```python
from build123d import *

# Parameters (mm, degrees)
AUFSATZ_LINEAR_AUSTRAGEN1_DEPTH = 25
VERRUNDUNG1_R                   = 0.2


with BuildPart() as part:
    # Skizze1 → Aufsatz-Linear austragen1 (new body)
    with BuildSketch(Plane.XY):
        Polygon((2.95, 2), (1, 2), (1, 0), (0, 0), (0, 2.79), (0.25, 2.79), (0.25, 3.01), (0, 3.01), (0, 5.8), (1, 5.8), (1, 3.8), (2.95, 3.8), align=None)
    extrude(amount=AUFSATZ_LINEAR_AUSTRAGEN1_DEPTH)

    # Verrundung1
    verrundung1_edges = [part.edges().sort_by_distance(p)[0] for p in [
        (0.5, 5.8, 0),
        (1, 4.8, 0),
        (0.25, 2.9, 25),
        (1.975, 3.8, 0),
        (2.95, 2.9, 0),
        (1.975, 2, 0),
        (1, 1, 0),
        (0.5, 0, 0),
        (0, 1.395, 0),
        (0.125, 2.79, 0),
        (0.25, 2.9, 0),
        (0.125, 3.01, 0),
        (0, 4.405, 0),
        (0.125, 2.79, 25),
        (0, 5.8, 12.5),
        (1, 5.8, 12.5),
        (0, 1.395, 25),
        (2.95, 3.8, 12.5),
        (2.95, 2, 12.5),
        (1, 0, 12.5),
        (0, 0, 12.5),
        (0.5, 0, 25),
        (1, 1, 25),
        (1.975, 2, 25),
        (2.95, 2.9, 25),
        (1.975, 3.8, 25),
        (1, 4.8, 25),
        (0.5, 5.8, 25),
        (0, 4.405, 25),
        (0.125, 3.01, 25),
    ]]
    fillet(verrundung1_edges, radius=VERRUNDUNG1_R)


solid = part.part
```
Geometry check sheet. Reference: the model listing, model coordinates, mm. A direction names the side the tool comes from. Give positions to 0.01 mm unless a question says otherwise; leave off trailing zeros. Write each loop counter-clockwise with the first axis right and the second up, starting at its lowest first coordinate (ties: lowest second). Pieces come first, ordered by that corner, then holes. Notation, with made-up numbers: (79.5, -15) -> (115.5, -15) arc R24 ccw to (115.5, -2) -> close; hole circle Ø1 at (75, 87). An arc over 180 degrees is marked (long way). Use one line per item in the form item = value.
Item 1: Access from +Z, -Z, +X, -X, +Y, -Y to the whole of each face (thin tool, end or side, straight path). Record for faces 1 (the flat face through (2.95, 3, 12)), 2 (the flat face through (1, 5, 12)), 3 (the flat face through (2, 2, 12)).
Results list:
face_1 = +Z, -Z, +X, +Y, -Y
face_2 = +Z, -Z, +X, +Y
face_3 = +Z, -Z, +X, -Y
Item 2: Depth check by flat-ended pin: pin 1 Ø0.9 at (x, z) = (2, 7.5) entering from -Y; pin 2 Ø2 at (y, z) = (4.5, 15.5) entering from +X; pin 3 Ø0.5 at (x, z) = (1.5, 9.5) entering from +Y; pin 4 Ø0.5 at (y, z) = (1, 13) entering from +X. Enter the tip coordinate at first touch or a pass-through.
Results list:
pin_1 = 2
pin_2 = 2.95
pin_3 = 3.8
pin_4 = 1
Item 3: Scan lines: line 1 (X direction, y = 1.15, z = 23.5); line 2 (Y direction, x = 1.1, z = 12); line 3 (Z direction, x = 0.9, y = 3.9). Record each from-to range of solid material in increasing order.
Results list:
line_1 = 0 to 1
line_2 = 2 to 3.8
line_3 = 0.03 to 24.97
Item 4: Sectioned sample at B-B on y = 5. Enter the section's corners in (x, z), plus the area to 3 significant figures.
Results list:
outline = (0, 0.2) arc R0.2 ccw to (0.2, 0) -> (0.8, 0) arc R0.2 ccw to (1, 0.2) -> (1, 24.8) arc R0.2 ccw to (0.8, 25) -> (0.2, 25) arc R0.2 ccw to (0, 24.8) -> close
area = 25.0 mm2
Item 5: Sectioned sample at C-C on z = 6.5. Enter the section's corners in (x, y), plus the area to 3 significant figures.
Results list:
outline = (0, 0.2) arc R0.2 ccw to (0.2, 0) -> (0.8, 0) arc R0.2 ccw to (1, 0.2) -> (1, 2) -> (2.75, 2) arc R0.2 ccw to (2.95, 2.2) -> (2.95, 3.6) arc R0.2 ccw to (2.75, 3.8) -> (1, 3.8) -> (1, 5.6) arc R0.2 ccw to (0.8, 5.8) -> (0.2, 5.8) arc R0.2 ccw to (0, 5.6) -> (0, 3.01) -> (0.25, 3.01) -> (0.25, 2.79) -> (0, 2.79) -> close
area = 9.20 mm2
Item 6: Sectioned sample at A-A on x = 1.6. Enter the section's corners in (y, z), plus the area to 3 significant figures.
Results list:
outline = (2, 0.2) arc R0.2 ccw to (2.2, 0) -> (3.6, 0) arc R0.2 ccw to (3.8, 0.2) -> (3.8, 24.8) arc R0.2 ccw to (3.6, 25) -> (2.2, 25) arc R0.2 ccw to (2, 24.8) -> close
area = 45.0 mm2
